Verification items for the finished model (mm, model axes). Face numbers are marked on the shaded views. A direction names the side the tool comes from. Round coordinates to 2 decimals unless told otherwise and drop trailing zeros. Loops run counter-clockwise (first coordinate to the right, second up) from the corner with the lowest first, then second, coordinate; pieces in that order, holes last. Notation, with made-up numbers: (61, -32.5) - (101, -32.5) arc R26 ccw to (101, -18.5) - close; hole circle Ø2 at (40.25, 25). An arc over 180 degrees is marked (long way). Use a Markdown table: item, result. Add a question column.
```python
from build123d import *

# Parameters (mm, degrees)
F0_W     = 406.4
F0_H     = 762
F1_DEPTH = 3.175
F2_W     = 406.4
F2_H     = 3.175
F3_DEPTH = 152.4
F4_W     = 3.175
F4_H     = 758.825
F5_DEPTH = 152.4
F6_W     = 403.225
F6_H     = 3.175
F7_DEPTH = 152.4
F8_W     = 3.175
F8_H     = 755.65
F9_DEPTH = 152.4


with BuildPart() as f1:
    # F0 (on Top) → F1 (new body)
    with BuildSketch(Plane.XY):
        Rectangle(F0_W, F0_H)
    extrude(amount=F1_DEPTH)

    # F2 (on face) → F3 (join)
    with BuildSketch(Plane.XY.offset(3.175)):
        with Locations((0, 379.4125)):
            Rectangle(F2_W, F2_H)
    extrude(amount=F3_DEPTH)

    # F4 (on face) → F5 (join)
    with BuildSketch(Plane.XY.offset(3.175)):
        with Locations((201.6125, -1.5875)):
            Rectangle(F4_W, F4_H)
    extrude(amount=F5_DEPTH)

    # F6 (on face) → F7 (join)
    with BuildSketch(Plane.XY.offset(3.175)):
        with Locations((-1.5875, -379.4125)):
            Rectangle(F6_W, F6_H)
    extrude(amount=F7_DEPTH)

    # F8 (on face) → F9 (join)
    with BuildSketch(Plane.XY.offset(3.175)):
        with Locations((-201.6125, 0)):
            Rectangle(F8_W, F8_H)
    extrude(amount=F9_DEPTH)


solid = f1.part
```
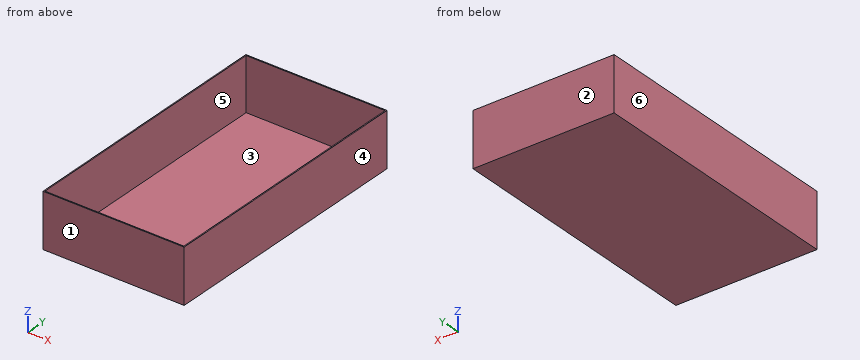
Q1. Set-up check for the marked faces 5 and 6: record each of +Z, -Z, +X, -X, +Y, -Y from which the full face is reachable in a straight line by a thin tool's end or side.
Q2. Section check C-C on x = -38. Record the cut outline in (y, z) (3 decimals), plus the area to 3 significant figures.
Q3. Go/stop test with a flat-tipped pin: pin 1 Ø5 at (x, y) = (-146.5, 144) entering from +Z (3 decimals). Record where the tip stops, or that it passes through.
Q4. Section check B-B on y = -313. Record the cut outline in (x, z) (3 decimals).
Q5. Section check A-A on z = 71. Record the cut outline in (x, y) (3 decimals).
Q6. Thickness scan on line 1 along X through (y, z) = (-120.5, 140.5) (3 decimals); line 2 along Y through (x, z) = (7, 7) (3 decimals); line 3 along Z through (x, y) = (10, 70.5) (3 decimals). Record the ranges inside material, lowest first.
Q7. Release check for a two-part mould opening along Y. For the marked faces 1, 2, 3 and 4 record: +Y half, -Y half, draft (parallel to the pull), parting line (faces both ways), or undercut.
Determined:
| question | item | result |
|---|---|---|
| 1 | face 5 | +Z |
| 1 | face 6 | +Z, -Z, -X, +Y, -Y |
| 2 | outline | (-381, 0) - (381, 0) - (381, 155.575) - (377.825, 155.575) - (377.825, 3.175) - (-377.825, 3.175) - (-377.825, 155.575) - (-381, 155.575) - close |
| 2 | area | 3,390 mm² |
| 3 | pin 1 | stops at z = 3.175 |
| 4 | outline | (-203.2, 0) - (203.2, 0) - (203.2, 155.575) - (200.025, 155.575) - (200.025, 3.175) - (-200.025, 3.175) - (-200.025, 155.575) - (-203.2, 155.575) - close |
| 5 | outline | (-203.2, -381) - (203.2, -381) - (203.2, 381) - (-203.2, 381) - close; hole (-200.025, -377.825) - (200.025, -377.825) - (200.025, 377.825) - (-200.025, 377.825) - close |
| 6 | line 1 | x = -203.2 to -200.025, 200.025 to 203.2 |
| 6 | line 2 | y = -381 to -377.825, 377.825 to 381 |
| 6 | line 3 | z = 0 to 3.175 |
| 7 | face 1 | -Y half |
| 7 | face 2 | +Y half |
| 7 | face 3 | undercut |
| 7 | face 4 | draft |
